Read the model definition and answer for the solid it produces. Units are mm, in the model's axes. A direction names the side the tool comes from. Round coordinates to 2 decimals unless told otherwise and drop trailing zeros. Order: outer loops, then holes, each group sorted by start corner. A loop starts at its lowest first (then second) coordinate and runs counter-clockwise, first axis right, second up. Notation, with made-up numbers: (33, 27) - (70, 27) arc R20 ccw to (70, 55) - close; hole circle Ø2 at (-32, -5). An arc over 180 degrees is marked (long way). Answer as a JSON object with one key per item and string values. Group by question number.
Q1. A tool of negligible diameter and unlimited length cuts with its end or side. For faces 1 (the flat face through (4, 15, 0)), 2 (the flat face through (5, 11.39, 59)), 3 (the flat face through (9, 3, -4.5)), from which of +Z, -Z, +X, -X, +Y, -Y can it reach the whole face along a straight path? Write none if from no direction.
Q2. Consider line 1 (Z direction, x = 2.5, y = 12.5); line 2 (Z direction, x = 5.75, y = 15.5); line 3 (Z direction, x = 9.25, y = 14.5). Determine where each line is inside the solid, lowest interval first.
Q3. A cutting plane is placed at A-A on z = -70. Determine the outline of the cut face in (x, y).
Q4. The mould has two halves that part along Y. Classify faces 4 (the flat face through (5, 2, -75)), 5 (the flat face through (5, 11.39, -59)), 6 (the cylindrical face through (5.07, 6.84, -58.57)): pulls with the +Y half, pulls with the -Y half, needs draft (parallel to the pull), parting line crosses it, or undercut.
Q5. Given pin 1 Ø2 at (x, y) = (3.5, 21) entering from +Z; pin 2 Ø3 at (x, z) = (4.5, -63.5) entering from +Y; pin 3 Ø4 at (x, y) = (4.5, 15) entering from -Z, each flat-ended and moving along its own axis, determine where each tip first touches the part or whether it passes through.
Q6. A cutting plane is placed at C-C on z = 22.5. Determine the outline of the cut face in (x, y), and give its area (3 significant figures).
Q7. A cutting plane is placed at B-B on z = -34.5. Determine the outline of the cut face in (x, y), and give its area (3 significant figures).
```python
from build123d import *

# Parameters (mm, degrees)
SKETCH_1_W          = 20
SKETCH_1_H          = 30
EXTRUDE_1_DEPTH     = 10
SKETCH_3_W          = 10
SKETCH_3_H          = 20
EXTRUDE_2_DEPTH     = 65
SKETCH_4_R          = 1.5
CUT_EXTRUDE_1_DEPTH = 78.136243103
SKETCH_5_W          = 9
SKETCH_5_H          = 30
CUT_EXTRUDE_2_DEPTH = 3
SKETCH_6_W          = 13
SKETCH_6_H          = 15
EXTRUDE_3_DEPTH     = 10
SKETCH_7_R          = 1.5
CUT_EXTRUDE_5_DEPTH = 121.841532616
SKETCH_8_W          = 20
SKETCH_8_H          = 20
CUT_EXTRUDE_6_DEPTH = 6.389884519


with BuildPart() as part:
    # 草图1 → 凸台-拉伸1 (new body)
    with BuildSketch(Plane(origin=(0, 0, 0), x_dir=(0, 0, -1), z_dir=(1, 0, 0))):
        Rectangle(SKETCH_1_W, SKETCH_1_H)
    extrude(amount=EXTRUDE_1_DEPTH)

    # 草图3 → 凸台-拉伸2 (add)
    with BuildSketch(Plane(origin=(0, 0, -10), x_dir=(-1, 0, 0), z_dir=(0, 0, -1))):
        with Locations((-5, 1.389884519)):
            Rectangle(SKETCH_3_W, SKETCH_3_H)
    extrude_2 = extrude(amount=EXTRUDE_2_DEPTH)

    # 镜向1: 凸台-拉伸2 across plane
    add(extrude_2.mirror(Plane.XY))

    # 草图4 → 切除-拉伸1 (cut, through all)
    with BuildSketch(Plane(origin=(10, 0, 0), x_dir=(0, 0, -1), z_dir=(1, 0, 0))):
        with Locations((-70, 6.389884519)):
            Circle(SKETCH_4_R)
        with Locations((-60, 6.389884519)):
            Circle(SKETCH_4_R)
        with Locations((-70, -3.610115481)):
            Circle(SKETCH_4_R)
        with Locations((-60, -3.610115481)):
            Circle(SKETCH_4_R)
    cut_extrude_1 = extrude(amount=-CUT_EXTRUDE_1_DEPTH, mode=Mode.SUBTRACT)

    # 镜向2: 切除-拉伸1 across plane
    add(cut_extrude_1.mirror(Plane.XY), mode=Mode.SUBTRACT)

    # 草图5 → 切除-拉伸2 (cut)
    with BuildSketch(Plane(origin=(10, 0, 0), x_dir=(0, 0, -1), z_dir=(1, 0, 0))):
        Rectangle(SKETCH_5_W, SKETCH_5_H)
    extrude(amount=-CUT_EXTRUDE_2_DEPTH, mode=Mode.SUBTRACT)

    # 草图6 → 凸台-拉伸3 (add)
    with BuildSketch(Plane(origin=(10, 0, 0), x_dir=(0, 0, -1), z_dir=(1, 0, 0))):
        with Locations((36, 18.889884519)):
            Rectangle(SKETCH_6_W, SKETCH_6_H)
        Polygon((10, 11.389884519), (19.5, 11.389884519), (19.5, 26.389884519), (10, 26.389884519), (10, 15), align=None)
    extrude_3 = extrude(amount=-EXTRUDE_3_DEPTH)

    # 草图7 → 切除-拉伸5 (cut, through all)
    with BuildSketch(Plane(origin=(0, 0, -42.5), x_dir=(-1, 0, 0), z_dir=(0, 0, -1))):
        with Locations((-5, 18.889884519)):
            Circle(SKETCH_7_R)
    cut_extrude_5 = extrude(amount=-CUT_EXTRUDE_5_DEPTH, mode=Mode.SUBTRACT)

    # 镜向4: 凸台-拉伸3, 切除-拉伸5 across plane
    add(extrude_3.mirror(Plane.XY))
    add(cut_extrude_5.mirror(Plane.XY), mode=Mode.SUBTRACT)

    # 草图8 → 切除-拉伸6 (cut)
    with BuildSketch(Plane.XZ.offset(15)):
        Rectangle(SKETCH_8_W, SKETCH_8_H)
    extrude(amount=-CUT_EXTRUDE_6_DEPTH, mode=Mode.SUBTRACT)


solid = part.part
```
Result set:
{
 "1": {"face 1": "+X, -X, +Y", "face 2": "+Z, +X, -X, +Y", "face 3": "+X, +Y, -Y"},
 "2": {"line 1": "z = -42.5 to -29.5, -19.5 to 19.5, 29.5 to 42.5", "line 2": "z = -42.5 to -29.5, -19.5 to -10, 10 to 19.5, 29.5 to 42.5", "line 3": "z = -42.5 to -29.5, -19.5 to -4.5, 4.5 to 19.5, 29.5 to 42.5"},
 "3": {"outline": "(0, -8.61) - (10, -8.61) - (10, -5.11) - (0, -5.11) - close; (0, -2.11) - (10, -2.11) - (10, 4.89) - (0, 4.89) - close; (0, 7.89) - (10, 7.89) - (10, 11.39) - (0, 11.39) - close"},
 "4": {"face 4": "needs draft", "face 5": "pulls with the +Y half", "face 6": "undercut"},
 "5": {"pin 1": "stops at z = 42.5", "pin 2": "stops at y = 11.39", "pin 3": "stops at z = -42.5"},
 "6": {"outline": "(0, -8.61) - (10, -8.61) - (10, 11.39) - (0, 11.39) - close", "area": "200 mm²"},
 "7": {"outline": "(0, -8.61) - (10, -8.61) - (10, 26.39) - (0, 26.39) - close; hole circle Ø3 at (5, 18.89)", "area": "343 mm²"}
}
